from build123d import *

# Parameters (mm, degrees)
SKETCH1_W           = 22.5
SKETCH1_H           = 11.9
BOSS_EXTRUDE1_DEPTH = 5
SKETCH2_R           = 1.5
BOSS_EXTRUDE2_DEPTH = 4


with BuildPart() as part:
    # Sketch1 → Boss-Extrude1 (new body, symmetric)
    with BuildSketch(Plane.XY):
        Rectangle(SKETCH1_W, SKETCH1_H)
    extrude(amount=BOSS_EXTRUDE1_DEPTH, both=True)

    # Sketch2 → Boss-Extrude2 (add)
    with BuildSketch(Plane(origin=(0, 0, -5), x_dir=(-1, 0, 0), z_dir=(0, 0, -1))):
        Circle(SKETCH2_R)
    extrude(amount=BOSS_EXTRUDE2_DEPTH)


solid = part.part
Work out the finished part from the listing and answer in its coordinate system (mm). A direction names the side the tool comes from. Give positions to 0.01 mm unless a question says otherwise; leave off trailing zeros. Write each loop counter-clockwise with the first axis right and the second up, starting at its lowest first coordinate (ties: lowest second). Pieces come first, ordered by that corner, then holes.
Q1. The part is cut by section A-A on x = 0. Give the vertices of the cut face in (y, z).
Answer:
outline: (-5.95, -5) - (-1.5, -5) - (-1.5, -9) - (1.5, -9) - (1.5, -5) - (5.95, -5) - (5.95, 5) - (-5.95, 5) - close
Q2. Straight lines are drawn through the part: L1, parallel to Z at x = -10, y = 4.5; L2, parallel to X at y = -0.5, z = -6.75; L3, parallel to Y at x = 0.25, z = -7.5. For each, find the intervals that lie inside material, in ascending order.
Answer:
L1: z = -5 to 5
L2: x = -1.41 to 1.41
L3: y = -1.48 to 1.48
Q3. A tool of negligible diameter and unlimited length cuts with its end or side. For faces 1 (the face through (11.25, 0, 0)), 2 (the face through (1.5, 0.07, -6.97)), from which of +Z, -Z, +X, -X, +Y, -Y can it reach the whole face along a straight path? Write none if from no direction.
Answer:
face 1: +Z, -Z, +X, +Y, -Y
face 2: -Z
Q4. The part is cut by section C-C on x = -8.5. Give the vertices of the cut face in (y, z), and give its area (3 significant figures).
Answer:
outline: (-5.95, -5) - (5.95, -5) - (5.95, 5) - (-5.95, 5) - close
area: 119 mm2
Q5. Given pin 1 (1 mm diameter, centred on x = 4, y = -0.5, fed in from -Z), flat-ended and moving along its own axis, determine where the tip first touches the part or whether it passes through.
Answer:
pin 1: stops at z = -5
Q6. The part is cut by section D-D on y = 5.25. Give the vertices of the cut face in (x, z), and give its area (3 significant figures).
Answer:
outline: (-11.25, -5) - (11.25, -5) - (11.25, 5) - (-11.25, 5) - close
area: 225 mm2
Q7. The part is cut by section B-B on y = 0. Give the vertices of the cut face in (x, z), and give its area (3 significant figures).
Answer:
outline: (-11.25, -5) - (-1.5, -5) - (-1.5, -9) - (1.5, -9) - (1.5, -5) - (11.25, -5) - (11.25, 5) - (-11.25, 5) - close
area: 237 mm2
